Work out the finished part from the listing and answer in its coordinate system (mm). A direction names the side the tool comes from. Coordinates: 2 decimals unless noted, no trailing zeros. Order: outer loops, then holes, each group sorted by start corner. A loop starts at its lowest first (then second) coordinate and runs counter-clockwise, first axis right, second up. Notation, with made-up numbers: M -32,2 L -14,2 A15 cw -14,8 Z; hole C 22,88 d4. An arc over 180 degrees is marked long. Use a Markdown table: item, result.
Autodesk Inventor part; units mm, degrees
ref_plane "YZ Plane" through (0, 0, 0) normal (1, 0, 0) x (0, 1, 0)
ref_plane "XZ Plane" through (0, 0, 0) normal (0, 1, 0) x (-1, 0, 0)
ref_plane "XY Plane" through (0, 0, 0) normal (0, 0, 1) x (1, 0, 0)
sketch "Sketch1" plane through (0, 0, 0) normal (0, 1, 0) x (-1, 0, 0)
  line L0 (27.5, -0.0615) -> (27.5, 89.9385)
  line L1 (-32.5, 89.9385) -> (-32.5, -0.0615)
  line L2 (-32.5, -0.0615) -> (-2.5, -0.0615)
  line L3 (-2.5, -0.0615) -> (-2.5, 89.9385) construction
  line L4 (-32.5, 44.9385) -> (-2.5, 44.9385) construction
  line L5 (-32.5, 89.9385) -> (27.5, 89.9385)
  line L6 (-21, 89.9385) -> (-9, 89.9385)
  line L7 (-9, 89.9385) -> (-9, 95.9385)
  line L8 (-9, 95.9385) -> (-21, 95.9385)
  line L9 (-21, 95.9385) -> (-21, 89.9385)
  line L10 (16, 89.9385) -> (4, 89.9385)
  line L11 (4, 89.9385) -> (4, 95.9385)
  line L12 (4, 95.9385) -> (16, 95.9385)
  line L13 (16, 95.9385) -> (16, 89.9385)
  line L14 (-2.5, 44.9385) -> (27.5, 44.9385) construction
  line L15 (-2.5, -0.0615) -> (27.5, -0.0615)
  line L16 (-9, 86.9385) -> (-21, 86.9385)
  line L17 (-21, 86.9385) -> (-21, 80.9385)
  line L18 (-21, 80.9385) -> (-9, 80.9385)
  line L19 (-9, 80.9385) -> (-9, 86.9385)
  line L20 (-9, 86.9385) -> (-21, 80.9385) construction
  line L21 (-21, 86.9385) -> (-9, 80.9385) construction
  line L22 (4, 86.9385) -> (16, 86.9385)
  line L23 (16, 86.9385) -> (16, 80.9385)
  line L24 (16, 80.9385) -> (4, 80.9385)
  line L25 (4, 80.9385) -> (4, 86.9385)
  line L26 (4, 86.9385) -> (16, 80.9385) construction
  line L27 (16, 86.9385) -> (4, 80.9385) construction
  point P0 (-15, 83.9385)
  point P1 (10, 83.9385)
  dimension "d0" = 60
  dimension "d1" = 90
  dimension "d18" = 12
  dimension "d19" = 6
  dimension "d20" = 18.5
  dimension "d21" = 12
  dimension "d22" = 6
  dimension "d23" = 3
extrude "Extrusion1" add sketch "Sketch1" along normal blind 6
sketch "Sketch2" plane through (0, 6, 0) normal (0, 1, 0) x (1, 0, 0)
  circle A0 centre (8, -19.9385) radius 1.4986
  circle A1 centre (27, -19.9385) radius 1.4986
  circle A2 centre (27, -36.4385) radius 1.4985
  circle A3 centre (8, -36.4385) radius 1.4985
  line L0 (27, -36.4385) -> (8, -36.4385) construction
  line L1 (8, -36.4385) -> (8, -19.9385) construction
  line L2 (8, -19.9385) -> (27, -19.9385) construction
  line L3 (27, -19.9385) -> (27, -36.4385) construction
  line L4 (27, -36.4385) -> (8, -19.9385) construction
  line L5 (27, -19.9385) -> (8, -36.4385) construction
  line L6 (32.5, 0.0615) -> (-27.5, 0.0615) construction
  line L7 (2.5, 0.0615) -> (2.5, -89.9385) construction
  line L8 (-4, -89.9385) -> (9, -89.9385) construction
  line L9 (-2.5, -49.9385) -> (-8.5, -49.9385)
  line L10 (-8.5, -49.9385) -> (-8.5, -43.9385)
  line L11 (-8.5, -43.9385) -> (-2.5, -43.9385)
  line L12 (-2.5, -43.9385) -> (-2.5, -49.9385)
  line L13 (-2.5, -28.9385) -> (-8.5, -28.9385)
  line L14 (-8.5, -28.9385) -> (-8.5, -22.9385)
  line L15 (-8.5, -22.9385) -> (-2.5, -22.9385)
  line L16 (-2.5, -22.9385) -> (-2.5, -28.9385)
  point P0 (0, 0)
  point P1 (17.5, -28.1885)
  dimension "d26" = 2.9972
  dimension "d28" = 2.9972
  dimension "d29" = 19
  dimension "d30" = 2.997
  dimension "d31" = 2.997
  dimension "d32" = 16.5
  dimension "d33" = 15
  dimension "d36" = 20
  dimension "d37" = 6
  dimension "d38" = 6
  dimension "d39" = 6
  dimension "d40" = 5
  dimension "d41" = 40
  dimension "d42" = 15
extrude "Extrusion2" cut sketch "Sketch2" against normal through all
properties part number "thumper-bumper-sidewall-v2"
1. Section A-A on x = 8 is taken. Determine the outline of the cut face in (y, z), then the cut area to 3 significant figures.
Answers below:
| item | result |
|---|---|
| outline | M 0,-0.06 L 6,-0.06 L 6,18.44 L 0,18.44 Z; M 0,21.44 L 6,21.44 L 6,34.94 L 0,34.94 Z; M 0,37.94 L 6,37.94 L 6,89.94 L 0,89.94 Z |
| area | 504 mm² |
2. For faces 1 (the face through (-16, 3, 93)), 2 (the face through (21, 3, 93)), 3 (the face through (-10, 3, 86.938)), determine the directions among +Z, -Z, +X, -X, +Y, -Y from which every point of the face is accessible in a straight line to the end or side of a thin tool.
Answers below:
| item | result |
|---|---|
| face 1 | +Z, -X, +Y, -Y |
| face 2 | +Z, +X, +Y, -Y |
| face 3 | +Y, -Y |
3. For a pull along Z with two mould halves and no side action, classify faces 4 (the face through (-6, 3, 22.938)), 5 (the face through (3, 3, -0.062)), 6 (the face through (3, 0, 49)) as +Z half, -Z half, draft (parallel to the pull), parting line (faces both ways), or undercut.
Answers below:
| item | result |
|---|---|
| face 4 | undercut |
| face 5 | -Z half |
| face 6 | draft |
4. A flat-ended cylindrical pin translates along its axis: P1, Ø2, axis at x = 7.5, y = 4.5, coming from the +Z side. Find the tip coordinate at first contact, or state that the pin passes through.
Answers below:
| item | result |
|---|---|
| P1 | z = 89.94 |
5. Find the intervals of material crossed by probe 1 along X at (y, z) = (4.5, 83); probe 2 along Z at (x, y) = (27, 3.6); probe 3 along Z at (x, y) = (12.5, 5.25), in increasing order.
Answers below:
| item | result |
|---|---|
| probe 1 | -27.5 to -16, -4 to 9, 21 to 32.5 |
| probe 2 | -0.06 to 18.44, 21.44 to 34.94, 37.94 to 89.94 |
| probe 3 | -0.06 to 80.94, 86.94 to 95.94 |
6. Section C-C on y = 4.45 is taken. Give the number of separate pieces and of enclosed holes in the cut face, then the cut area to 3 significant figures.
Answers below:
| item | result |
|---|---|
| separate pieces | 1 |
| enclosed holes | 8 |
| area | 5,300 mm² |
7. Section B-B on x = -10 is taken. Determine the outline of the cut face in (y, z).
Answers below:
| item | result |
|---|---|
| outline | M 0,-0.06 L 6,-0.06 L 6,80.94 L 0,80.94 Z; M 0,86.94 L 6,86.94 L 6,95.94 L 0,95.94 Z |
